from build123d import *

# Parameters (mm, degrees)
F1_DEPTH = 12.7
F2_R     = 1.58749
F3_R     = 1.5875
F5_D     = 4.4958


# Not quite as in the source:
# - a fillet or chamfer is up to 0.001 mm smaller than in the source, because OpenCascade refuses the exact size


with BuildPart() as f1:
    # F0 (on Top) → F1 (new body, symmetric)
    with BuildSketch(Plane.XY):
        with BuildLine():
            Line((0, 43.3605122421), (0, 0))
            ThreePointArc((0, 0), (-29.1569779212, -8.6950956004), (-9.525, 14.5496778315))
            Line((-9.525, 14.5496778315), (-9.525, 17.9605122421))
            ThreePointArc((-9.525, 17.9605122421), (-31.4292598667, -10.9985226281), (3.175, 0))
            Line((3.175, 0), (3.175, 43.3605122421))
            Line((3.175, 43.3605122421), (0, 43.3605122421))
        make_face()
    extrude(amount=F1_DEPTH, both=True)

    # F2 (radius 1.5875 in the source; OpenCascade refuses exactly that, so slightly less here)
    f2_edges = [f1.edges().sort_by_distance(p)[0] for p in [
        (-9.525, 14.549678, 0),
        (-9.525, 17.960512, 0),
    ]]
    fillet(f2_edges, radius=F2_R)

    # F3
    f3_edges = [f1.edges().sort_by_distance(p)[0] for p in [
        (1.5875, 43.360512, 12.7),
        (1.5875, 43.360512, -12.7),
    ]]
    fillet(f3_edges, radius=F3_R)

    # F5 (through all)
    with Locations(Plane(origin=(0, 0, 0), x_dir=(0, 1, 0), z_dir=(-1, 0, 0))):
        with Locations((33.8355122421, 0)):
            Hole(F5_D / 2)


solid = f1.part
Here's how the part is built. I have some questions about the finished solid (model axes, mm). A direction names the side the tool comes from. Round coordinates to 2 decimals unless told otherwise and drop trailing zeros. Write each loop counter-clockwise with the first axis right and the second up, starting at its lowest first coordinate (ties: lowest second). Pieces come first, ordered by that corner, then holes.
1. For faces 1 (the cylindrical face through (-10.139, 15.547, 0.178)), 2 (the cylindrical face through (1.57, 42.88, 12.25)), 3 (the cylindrical face through (-9.855, 17.769, 0.178)), which set-ups out of +Z, -Z, +X, -X, +Y, -Y let a thin tool reach every point of the face, with its end or its side?
2. I need wall thicknesses on L1, parallel to X at y = 0, z = -0.25 (3 decimals); L2, parallel to X at y = 34.5, z = -5.75 (3 decimals); L3, parallel to X at y = -2, z = 1.75. Which ranges of each line are inside material? Lowest first, please.
3. Will these pins go through, and if not, where does the flat tip stop? pin 1 Ø5 at (y, z) = (33.84, 0) entering from -X; pin 2 Ø2 at (y, z) = (-10, 2) entering from +X; pin 3 Ø1.5 at (x, z) = (-29, 9) entering from -Y.
4. Suppose I cut it at B-B (x = -18). List the corners of the cut face in (y, z) for me.
5. Suppose I cut it at D-D (y = 23). List the corners of the cut face in (x, z) for me (3 decimals).
6. Suppose I cut it at C-C (y = 9). List the corners of the cut face in (x, z) for me (3 decimals).
7. If we mould it in two halves opening along Y, with no side actions, what happens to faces 4 (the cylindrical face through (-28.197, -10.009, 0.178)), 5 (the cylindrical face through (1.61, 31.76, 0.86)), 6 (the flat face through (0, 22, 0)), 7 (the flat face through (2, 43.361, 0))? For each: released by +Y, released by -Y, zero draft, split by the parting line, or undercut.
Answer sheet:
1. face 1: +Z, -Z
1. face 2: +Z, +X, -X, +Y
1. face 3: +Z, -Z, +Y
2. L1: x = -34.925 to -31.75, 0 to 3.175
2. L2: x = 0 to 3.175
2. L3: x = -34.82 to -31.62, -0.13 to 3.07
3. pin 1: stops at x = 0
3. pin 2: stops at x = 0.91
3. pin 3: stops at y = -14.48
4. outline: (-18.93, -12.7) - (-15.73, -12.7) - (-15.73, 12.7) - (-18.93, 12.7) - close; (15.73, -12.7) - (18.93, -12.7) - (18.93, 12.7) - (15.73, 12.7) - close
5. outline: (0, -12.7) - (3.175, -12.7) - (3.175, 12.7) - (0, 12.7) - close
6. outline: (-32.665, -12.7) - (-28.952, -12.7) - (-28.952, 12.7) - (-32.665, 12.7) - close; (0, -12.7) - (3.175, -12.7) - (3.175, 12.7) - (0, 12.7) - close
7. face 4: undercut
7. face 5: undercut
7. face 6: zero draft
7. face 7: released by +Y
